```python
from build123d import *

# Parameters (mm, degrees)
SKETCH1_R                = 111
SKETCH1_R_2              = 103.25
BOSS_EXTRUDE1_DEPTH      = 3.175
SKETCH1_R_3              = 53.45
SKETCH1_R_4              = 44.45
BOSS_EXTRUDE1_2_DEPTH    = 3.175
BOSS_EXTRUDE2_DEPTH      = 6.35
FILLET1_R                = 3.125
CIRPATTERN2_COUNT        = 6
FILLET1_OF_CIRPATTERN2_R = 3.125
M3_CLEARANCE_HOLE1_D     = 3.4
CIRPATTERN3_COUNT        = 8
SKETCH5_R                = 1.7
CUT_EXTRUDE1_DEPTH       = 1
CUT_EXTRUDE1_DEPTH_BACK  = 7.35
CUT_EXTRUDE6_DEPTH       = 4
M3_CLEARANCE_HOLE2_D     = 3.4
M3_CLEARANCE_HOLE3_D     = 3.2
M3X0_5_TAPPED_HOLE1_D    = 2.5


with BuildPart() as part:
    # Sketch1 → Boss-Extrude1 (new body, symmetric)
    with BuildSketch(Plane.XY):
        Circle(SKETCH1_R)
        Circle(SKETCH1_R_2, mode=Mode.SUBTRACT)
    extrude(amount=BOSS_EXTRUDE1_DEPTH, both=True)



with BuildPart() as body_2:
    # Sketch1 → Boss-Extrude1 2 (new body, symmetric)
    with BuildSketch(Plane.XY):
        Circle(SKETCH1_R_3)
        Circle(SKETCH1_R_4, mode=Mode.SUBTRACT)
    extrude(amount=BOSS_EXTRUDE1_2_DEPTH, both=True)


with BuildPart() as part_1:
    add(part.part)

    add(body_2.part)  # Boss-Extrude2 merges body 2
    # Sketch2 → Boss-Extrude2 (add, through all)
    with BuildSketch(Plane.XY.offset(3.175)):
        with BuildLine():
            Line((3.75, -103.181878254), (3.75, -53.318289545))
            ThreePointArc((3.75, -53.318289545), (0, -53.45), (-3.75, -53.318289545))
            Line((-3.75, -53.318289545), (-3.75, -103.181878254))
            ThreePointArc((-3.75, -103.181878254), (0, -103.25), (3.75, -103.181878254))
        make_face()
    boss_extrude2 = extrude(amount=-BOSS_EXTRUDE2_DEPTH)

    # Fillet1
    fillet1_edges = [part_1.edges().sort_by_distance(p)[0] for p in [
        (-3.75, -53.318289545, 0),
        (3.75, -53.318289545, 0),
        (3.75, -103.181878254, 0),
        (-3.75, -103.181878254, 0),
    ]]
    fillet(fillet1_edges, radius=FILLET1_R)

    # CirPattern2: Boss-Extrude2 ×6 about axis
    cirpattern2_axis = Axis((0, 0, 0), (0, 0, 1))
    for i in range(1, CIRPATTERN2_COUNT):
        add(boss_extrude2.rotate(cirpattern2_axis, i * 360 / CIRPATTERN2_COUNT))

    # Fillet1 of CirPattern2
    fillet1_of_cirpattern2_edges = [part_1.edges().sort_by_distance(p)[0] for p in [
        (44.299993232, -29.906740037, 0),
        (48.049993232, -23.411549508, 0),
        (91.233127778, -48.343343863, 0),
        (87.483127778, -54.838534391, 0),
        (48.049993232, 23.411549508, 0),
        (44.299993232, 29.906740037, 0),
        (87.483127778, 54.838534391, 0),
        (91.233127778, 48.343343863, 0),
        (3.75, 53.318289545, 0),
        (-3.75, 53.318289545, 0),
        (-3.75, 103.181878254, 0),
        (3.75, 103.181878254, 0),
        (-44.299993232, 29.906740037, 0),
        (-48.049993232, 23.411549508, 0),
        (-91.233127778, 48.343343863, 0),
        (-87.483127778, 54.838534391, 0),
        (-48.049993232, -23.411549508, 0),
        (-44.299993232, -29.906740037, 0),
        (-87.483127778, -54.838534391, 0),
        (-91.233127778, -48.343343863, 0),
    ]]
    fillet(fillet1_of_cirpattern2_edges, radius=FILLET1_OF_CIRPATTERN2_R)

    # M3 Clearance Hole1 (through all)
    with Locations(Plane.XY.offset(3.175)):
        with Locations((0, 107.125)):
            m3_clearance_hole1 = Hole(M3_CLEARANCE_HOLE1_D / 2)

    # CirPattern3: M3 Clearance Hole1 ×8 about axis
    cirpattern3_axis = Axis((0, 0, 0), (0, 0, 1))
    for i in range(1, CIRPATTERN3_COUNT):
        add(m3_clearance_hole1.rotate(cirpattern3_axis, i * 360 / CIRPATTERN3_COUNT), mode=Mode.SUBTRACT)

    # Sketch5 → Cut-Extrude1 (cut, two sides)
    with BuildSketch(Plane(origin=(0, 0, -3.175), x_dir=(-1, 0, 0), z_dir=(0, 0, -1))) as cut_extrude1_sk:
        with BuildLine():
            Line((53.376748633, -2.797356861), (44.38908282, -2.326333255))
            ThreePointArc((44.38908282, -2.326333255), (0, -44.45), (-44.38908282, -2.326333255))
            Line((-44.38908282, -2.326333255), (-53.376748633, -2.797356861))
            ThreePointArc((-53.376748633, -2.797356861), (-52.077963884, -12.032795921), (-49.193633081, -20.901889013))
            ThreePointArc((-49.193633081, -20.901889013), (-49.106095125, -23.114991521), (-50.507280946, -24.830265231))
            Line((-50.507280946, -24.830265231), (-88.3811414, -46.69674876))
            ThreePointArc((-88.3811414, -46.69674876), (-90.855666768, -46.979371485), (-92.750871157, -45.363403748))
            ThreePointArc((-92.750871157, -45.363403748), (-99.947075975, -25.906456802), (-103.108499463, -5.403687482))
            Line((-103.108499463, -5.403687482), (-110.847878358, -5.809291143))
            ThreePointArc((-110.847878358, -5.809291143), (0, -111), (110.847878358, -5.809291143))
            Line((110.847878358, -5.809291143), (103.108499463, -5.403687482))
            ThreePointArc((103.108499463, -5.403687482), (99.947075975, -25.906456802), (92.750871157, -45.363403748))
            ThreePointArc((92.750871157, -45.363403748), (90.855666768, -46.979371485), (88.3811414, -46.69674876))
            Line((88.3811414, -46.69674876), (50.507280946, -24.830265231))
            ThreePointArc((50.507280946, -24.830265231), (49.106095125, -23.114991521), (49.193633081, -20.901889013))
            ThreePointArc((49.193633081, -20.901889013), (52.077963884, -12.032795921), (53.376748633, -2.797356861))
        make_face()
        with Locations((-75.748813935, -75.748813935)):
            Circle(SKETCH5_R, mode=Mode.SUBTRACT)
        with Locations((0, -107.125)):
            Circle(SKETCH5_R, mode=Mode.SUBTRACT)
        with BuildLine():
            ThreePointArc((-46.757280946, -31.32545576), (-44.571217428, -30.969630098), (-42.698383412, -32.151991446))
            ThreePointArc((-42.698383412, -32.151991446), (-26.725, -46.289057832), (-6.495249669, -53.053880459))
            ThreePointArc((-6.495249669, -53.053880459), (-4.534877697, -54.084621619), (-3.75, -56.155720991))
            Line((-3.75, -56.155720991), (-3.75, -99.888688048))
            ThreePointArc((-3.75, -99.888688048), (-4.742504224, -102.173001242), (-7.089575531, -103.006312519))
            ThreePointArc((-7.089575531, -103.006312519), (-51.625, -89.417122941), (-85.661295626, -57.642908771))
            ThreePointArc((-85.661295626, -57.642908771), (-86.113162544, -55.193629757), (-84.6311414, -53.191939288))
            Line((-84.6311414, -53.191939288), (-46.757280946, -31.32545576))
        make_face(mode=Mode.SUBTRACT)
        with BuildLine():
            ThreePointArc((84.6311414, -53.191939288), (86.113162544, -55.193629757), (85.661295626, -57.642908771))
            ThreePointArc((85.661295626, -57.642908771), (51.625, -89.417122941), (7.089575531, -103.006312519))
            ThreePointArc((7.089575531, -103.006312519), (4.742504224, -102.173001242), (3.75, -99.888688048))
            Line((3.75, -99.888688048), (3.75, -56.155720991))
            ThreePointArc((3.75, -56.155720991), (4.534877697, -54.084621619), (6.495249669, -53.053880459))
            ThreePointArc((6.495249669, -53.053880459), (26.725, -46.289057832), (42.698383412, -32.151991446))
            ThreePointArc((42.698383412, -32.151991446), (44.571217428, -30.969630098), (46.757280946, -31.32545576))
            Line((46.757280946, -31.32545576), (84.6311414, -53.191939288))
        make_face(mode=Mode.SUBTRACT)
        with Locations((75.748813935, -75.748813935)):
            Circle(SKETCH5_R, mode=Mode.SUBTRACT)
    extrude(amount=CUT_EXTRUDE1_DEPTH, mode=Mode.SUBTRACT)
    extrude(cut_extrude1_sk.sketch, amount=-CUT_EXTRUDE1_DEPTH_BACK, mode=Mode.SUBTRACT)

    # Sketch6 → Cut-Extrude6 (cut)
    with BuildSketch(Plane.XY):
        Polygon((0, 0), (199.725906951, 10.467191249), (199.725906951, -44.207372647), align=None)
    cut_extrude6 = extrude(amount=-CUT_EXTRUDE6_DEPTH, mode=Mode.SUBTRACT)

    # Mirror1: Cut-Extrude6 across plane
    add(cut_extrude6.mirror(Plane(origin=(0, 0, 0), x_dir=(0, 0, 1), z_dir=(1, 0, 0))), mode=Mode.SUBTRACT)

    # M3 Clearance Hole2 (through all)
    with Locations(Plane.XY.offset(3.175)):
        with Locations((-49, 0)):
            Hole(M3_CLEARANCE_HOLE2_D / 2)

    # M3 Clearance Hole3 (through all)
    with Locations(Plane.XY.offset(3.175)):
        with Locations((49, 0)):
            Hole(M3_CLEARANCE_HOLE3_D / 2)

    # M3x0.5 Tapped Hole1 (through all)
    with Locations(Plane(origin=(0, 0, -3.175), x_dir=(-1, 0, 0), z_dir=(0, 0, -1))):
        with Locations((-9.336558942, 106.717357033), (-94.29157403, 50.841564609), (-44.010069559, 23.730018487), (-4.357787137, 49.809734905), (4.357787137, 49.809734905), (44.010069559, 23.730018487), (94.29157403, 50.841564609), (9.336558942, 106.717357033)):
            Hole(M3X0_5_TAPPED_HOLE1_D / 2)


solid = part_1.part
```
CAD build for the part. Positions are in the model's coordinates, mm. A direction names the side the tool comes from. Round coordinates to 2 decimals unless told otherwise and drop trailing zeros. Write each loop counter-clockwise with the first axis right and the second up, starting at its lowest first coordinate (ties: lowest second). Pieces come first, ordered by that corner, then holes. Notation, with made-up numbers: (73.25, -33) - (95.25, -33) arc R27 ccw to (95.25, 6) - close; hole circle Ø1 at (3.25, -35). An arc over 180 degrees is marked (long way). Write item = value, one per line. Start each with the question number.
Q1. Band-saw the part on C-C (y = 12.5). Give the cut face in (x, z) (3 decimals).
Q2. Mould opens along X. For faces 1 (the cylindrical face through (101.24, 20.28, -0.04)), 2 (the flat face through (51, 0, 0)), 3 (the cylindrical face through (1.01, 44.44, -0.04)), 4 (the cylindrical face through (2.52, 110.97, 0.04)) say: pulls with the +X half, pulls with the -X half, needs draft (parallel to the pull), parting line crosses it, or undercut.
Q3. Band-saw the part on A-A (y = 71.5). Give the cut face in (x, z) (3 decimals).
Q4. Band-saw the part on B-B (x = 32.5). Give the cut face in (y, z) (3 decimals), then the cut area to 3 significant figures.
Q5. Drop flat-ended pins along their axis: pin 1 (2 mm diameter, centred on x = -4.36, y = 49.81, fed in from -Z); pin 2 (4 mm diameter, centred on x = -106.5, y = -2.5, fed in from -Z); pin 3 (4 mm diameter, centred on x = -44.01, y = 23.73, fed in from -Z) (3 decimals); pin 4 (3 mm diameter, centred on y = 68, z = 0.5, fed in from +X). Give the stop position or say it passes through.
Q6. Probe L1, parallel to X at y = 48.5, z = 2.5; L2, parallel to Y at x = -75, z = 1.75; L3, parallel to X at y = 73, z = 0.25. List the from-to ranges inside material, lowest first. Write a range as from..to.
Q7. Band-saw the part on D-D (z = -1.25). Count the separate pieces of the cut face and the enclosed holes in it, then the cut area to 3 significant figures.
Q8. Which spindle directions (+Z, -Z, +X, -X, +Y, -Y) get a long thin tool onto all of the face, cutting with end or side? Do faces 5 (the cylindrical face through (-49.1, 23.1, 0)), 6 (the flat face through (-1, 53, 3.175)). Say none if no direction does.
Answers below:
q1.outline = (-110.294, -3.175) - (-102.491, -3.175) - (-102.491, 3.175) - (-110.294, 3.175) - close; (-51.968, -3.175) - (-42.656, -3.175) - (-42.656, 3.175) - (-51.968, 3.175) - close; (42.656, -3.175) - (51.968, -3.175) - (51.968, 3.175) - (42.656, 3.175) - close; (102.491, -3.175) - (110.294, -3.175) - (110.294, 3.175) - (102.491, 3.175) - close
q2.face_1 = undercut
q2.face_2 = needs draft
q2.face_3 = undercut
q2.face_4 = parting line crosses it
q3.outline = (-84.904, -3.175) - (-74.487, -3.175) - (-74.487, 3.175) - (-84.904, 3.175) - close; (-3.75, -3.175) - (3.75, -3.175) - (3.75, 3.175) - (-3.75, 3.175) - close; (74.487, -3.175) - (84.904, -3.175) - (84.904, 3.175) - (74.487, 3.175) - close
q4.outline = (30.324, -3.175) - (42.434, -3.175) - (42.434, 3.175) - (30.324, 3.175) - close; (98.002, -3.175) - (106.136, -3.175) - (106.136, 3.175) - (98.002, 3.175) - close
q4.area = 129 mm2
q5.pin_1 = through
q5.pin_2 = 0
q5.pin_3 = -3.175
q5.pin_4 = 88.87
q6.L1 = -99.84..-76.5, -22.46..22.46, 76.5..99.84
q6.L2 = 38.97..47.63, 70.96..74.22, 77.28..81.83
q6.L3 = -83.62..-73.02, -3.75..3.75, 73.02..83.62
q7.separate_pieces = 1
q7.enclosed_holes = 13
q7.area = 4,940 mm2
q8.face_5 = +Z, -Z
q8.face_6 = +Z, +X, -X, +Y, -Y
